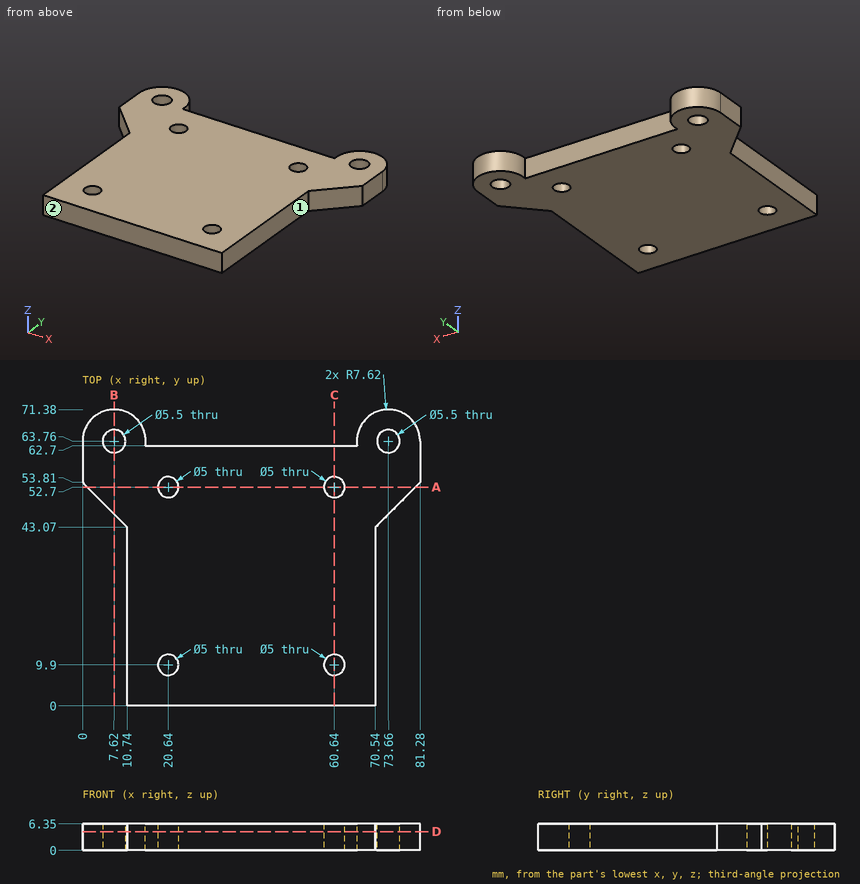
Source: three-view drawing plus pictorial views. Frame: mm from the lowest corner of the part. A direction names the side the tool comes from. Round coordinates to 2 decimals unless told otherwise and drop trailing zeros. Write each loop counter-clockwise with the first axis right and the second up, starting at its lowest first coordinate (ties: lowest second). Pieces come first, ordered by that corner, then holes. Notation, with made-up numbers: M -28.75,-35 L 14.25,-35 A18 cw 14.25,-5 Z; hole C 77,27.5 d10. An arc over 180 degrees is marked long. One line per item, written item: value. Start each with the question number.
Item 1: Section query B-B (x = 7.62). Return the cut outline in (y, z).
Item 2: Section query C-C (x = 60.64). Return the cut outline in (y, z).
Item 3: Pin query (flat end, axial travel): pin 1 (1.5 mm diameter, centred on x = 57, z = 1, fed in from +Y); pin 2 (3 mm diameter, centred on y = 13.5, z = 1.5, fed in from +X); pin 3 (2 mm diameter, centred on y = 19.5, z = 2, fed in from -X). Return the tip coordinate at first contact, or that it passes through.
Item 4: Set-up query: the marked faces 1 and 2. Return all of +Z, -Z, +X, -X, +Y, -Y with unobstructed straight access to the full face (end or side cutting, diameter ignored); none if empty.
Item 5: Section query D-D (z = 4.5). Return the cut outline in (x, y).
Item 6: Ray query, L1, parallel to Y at x = 20.64, z = 1.5; L2, parallel to X at y = 64, z = 4.5; L3, parallel to X at y = 61.5, z = 4.5. Return the intervals inside material, ascending. Write a range as from..to.
Item 7: Section query A-A (y = 52.7). Return the cut outline in (x, z), plus the area to 3 significant figures.
Result set:
1. outline: M 46.19,0 L 61.01,0 L 61.01,6.35 L 46.19,6.35 Z; M 66.51,0 L 71.38,0 L 71.38,6.35 L 66.51,6.35 Z
2. outline: M 0,0 L 7.4,0 L 7.4,6.35 L 0,6.35 Z; M 12.4,0 L 50.2,0 L 50.2,6.35 L 12.4,6.35 Z; M 55.2,0 L 62.7,0 L 62.7,6.35 L 55.2,6.35 Z
3. pin 1: stops at y = 62.7
3. pin 2: stops at x = 70.54
3. pin 3: stops at x = 10.74
4. face 1: +Z, -Z, +X, -Y
4. face 2: +Z, -Z, +X, -X, -Y
5. outline: M 0,53.81 L 10.74,43.07 L 10.74,0 L 70.54,0 L 70.54,43.07 L 81.28,53.81 L 81.28,63.76 A7.62 ccw long 66.11,62.7 L 15.17,62.7 A7.62 ccw long 0,63.76 Z; hole C 7.62,63.76 d5.5; hole C 20.64,9.9 d5; hole C 20.64,52.7 d5; hole C 60.64,9.9 d5; hole C 60.64,52.7 d5; hole C 73.66,63.76 d5.5
6. L1: y = 0..7.4, 12.4..50.2, 55.2..62.7
6. L2: x = 0..4.88, 10.36..15.24, 66.04..70.92, 76.4..81.28
6. L3: x = 0..6.05, 9.19..72.09, 75.23..81.28
7. outline: M 1.11,0 L 18.14,0 L 18.14,6.35 L 1.11,6.35 Z; M 23.14,0 L 58.14,0 L 58.14,6.35 L 23.14,6.35 Z; M 63.14,0 L 80.17,0 L 80.17,6.35 L 63.14,6.35 Z
7. area: 439 mm²
